```python
from build123d import *

# Parameters (mm, degrees)
BOSS_EXTRUDE1_DEPTH = 1
BOSS_EXTRUDE2_DEPTH = 1


with BuildPart() as part:
    # Sketch1 → Boss-Extrude1 (new body)
    with BuildSketch(Plane(origin=(0, 0, 0), x_dir=(1, 0, 0), z_dir=(0, 1, 0))):
        with BuildLine():
            Line((-3, 4), (3, 4))
            ThreePointArc((3, 4), (5, 0), (3, -4))
            Line((3, -4), (-3, -4))
            ThreePointArc((-3, -4), (-5, 0), (-3, 4))
        make_face()
    extrude(amount=BOSS_EXTRUDE1_DEPTH)

    # Sketch2 → Boss-Extrude2 (add)
    with BuildSketch(Plane(origin=(0, 1, 0), x_dir=(1, 0, 0), z_dir=(0, 1, 0))):
        with BuildLine():
            Line((4, 0.5), (4, -0.5))
            Line((4, -0.5), (4.974937186, -0.5))
            ThreePointArc((4.974937186, -0.5), (5, 0), (4.974937186, 0.5))
            Line((4.974937186, 0.5), (4, 0.5))
        make_face()
        with BuildLine():
            Line((-4, -0.5), (-4, 0.5))
            Line((-4, 0.5), (-4.974937186, 0.5))
            ThreePointArc((-4.974937186, 0.5), (-5, 0), (-4.974937186, -0.5))
            Line((-4.974937186, -0.5), (-4, -0.5))
        make_face()
    extrude(amount=BOSS_EXTRUDE2_DEPTH)


solid = part.part
```
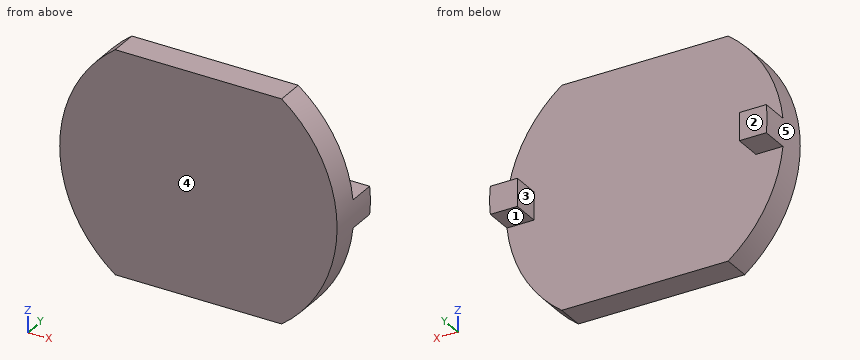
Can you work these out from the model? Positions are in its coordinate system, mm. Face numbers are marked on the shaded views. A direction names the side the tool comes from. Round coordinates to 2 decimals unless told otherwise and drop trailing zeros. Loops run counter-clockwise (first coordinate to the right, second up) from the corner with the lowest first, then second, coordinate; pieces in that order, holes last. Notation, with made-up numbers: M 59,15 L 97,15 A37 ccw 97,54 Z; hole C 81,51 d7. An arc over 180 degrees is marked long. Write item = value, one per line. Start each with the question number.
(1) Suppose I cut it at B-B on z = 0.25. Write out the boundary of the cut face in (x, y), plus the area to 3 significant figures.
(2) Suppose I cut it at D-D on y = 0.85. Write out the boundary of the cut face in (x, z).
(3) If we mould it in two halves opening along X, with no side actions, what happens to the marked faces 3, 4 and 5? For each: released by +X, released by -X, zero draft, split by the parting line, or undercut.
(4) Suppose I cut it at C-C on x = 2.5. Write out the boundary of the cut face in (y, z), plus the area to 3 significant figures.
(5) I need wall thicknesses on line 1 along X through (y, z) = (1.5, 0); line 2 along Y through (x, z) = (-2, -0.25); line 3 along X through (y, z) = (0.1, -3). Which ranges of each line are inside material? Lowest first, please.
(6) Which directions (+Z, -Z, +X, -X, +Y, -Y) give clear straight access to the entire face, cutting with the end or side of a thin tool? Please do the marked faces 1 and 2.
(7) I'm going to push flat-ended pins straight in: P1, Ø1, axis at x = 3, z = 0, coming from the +Y side; P2, Ø1, axis at y = 0.5, z = 1, coming from the +X side; P3, Ø0.8, axis at x = 4.5, y = 1.5, coming from the -Z side. Where does each tip first touch, or does it pass through?
(8) Suppose I cut it at A-A on y = 1.4. Write out the boundary of the cut face in (x, z).
Answer block:
q1.outline = M -4.99,0 L 4.99,0 L 4.99,2 L 4,2 L 4,1 L -4,1 L -4,2 L -4.99,2 Z
q1.area = 12.0 mm²
q2.outline = M -3,-4 L 3,-4 A5 ccw 3,4 L -3,4 A5 ccw Z
q3.face_3 = undercut
q3.face_4 = zero draft
q3.face_5 = released by -X
q4.outline = M 0,-4 L 1,-4 L 1,4 L 0,4 Z
q4.area = 8.00 mm²
q5.line_1 = -5 to -4, 4 to 5
q5.line_2 = 0 to 1
q5.line_3 = -4 to 4
q6.face_1 = -Z, +X, -X, +Y
q6.face_2 = +Z, -Z, +X, -X, +Y
q7.P1 = 1
q7.P2 = 4.97
q7.P3 = -0.5
q8.outline = M -4.97,-0.5 L -4,-0.5 L -4,0.5 L -4.97,0.5 A5 ccw Z; M 4,-0.5 L 4.97,-0.5 A5 ccw 4.97,0.5 L 4,0.5 Z
